Check sheet for the modelled part. Datum: model origin and axes. Units: mm. Face numbers are marked on the shaded views. A direction names the side the tool comes from. Coordinates: 2 decimals unless noted, no trailing zeros. Loops run counter-clockwise (first coordinate to the right, second up) from the corner with the lowest first, then second, coordinate; pieces in that order, holes last. Notation, with made-up numbers: M 2,-8.5 L 27,-8.5 A31 ccw 27,18.5 Z; hole C 82,44 d1. An arc over 180 degrees is marked long. Write each question's results on one line, items separated by ' | '. Start each with the question number.
from build123d import *

# Parameters (mm, degrees)
SKETCH1_W           = 32
SKETCH1_H           = 46
BOSS_EXTRUDE1_DEPTH = 25.2
BOSS_EXTRUDE2_START = 25.2
BOSS_EXTRUDE2_DEPTH = 16.5
SKETCH2_R           = 12.2
BOSS_EXTRUDE3_DEPTH = 30.8


with BuildPart() as part:
    # Sketch1 → Boss-Extrude1 (new body)
    # profile 1 of 2: a face of its own
    with BuildSketch(Plane(origin=(0, 0, 0), x_dir=(1, 0, 0), z_dir=(0, 1, 0))):
        with Locations((0, -8)):
            Rectangle(SKETCH1_W, SKETCH1_H)
        with BuildLine():
            ThreePointArc((-1.8, 2.4), (0, -3), (1.8, 2.4))
            Line((1.8, 2.4), (-1.8, 2.4))
        make_face(mode=Mode.SUBTRACT)
    # profile 2 of 2: a face of its own
    with BuildSketch(Plane(origin=(0, 0, 0), x_dir=(1, 0, 0), z_dir=(0, 1, 0))):
        with BuildLine():
            Line((-1.8, 2.4), (1.8, 2.4))
            ThreePointArc((1.8, 2.4), (0, -3), (-1.8, 2.4))
        make_face()
    extrude(amount=BOSS_EXTRUDE1_DEPTH)

    # Sketch1<3> → Boss-Extrude2 (add)
    with BuildSketch(Plane(origin=(0, 0, 0), x_dir=(1, 0, 0), z_dir=(0, 1, 0)).offset(BOSS_EXTRUDE2_START)):
        with BuildLine():
            Line((-1.8, 2.4), (1.8, 2.4))
            ThreePointArc((1.8, 2.4), (0, -3), (-1.8, 2.4))
        make_face()
    extrude(amount=BOSS_EXTRUDE2_DEPTH)

    # Sketch2 → Boss-Extrude3 (add)
    with BuildSketch(Plane.XY.offset(31)):
        with Locations((3.8, 13)):
            Circle(SKETCH2_R)
    extrude(amount=BOSS_EXTRUDE3_DEPTH)


solid = part.part
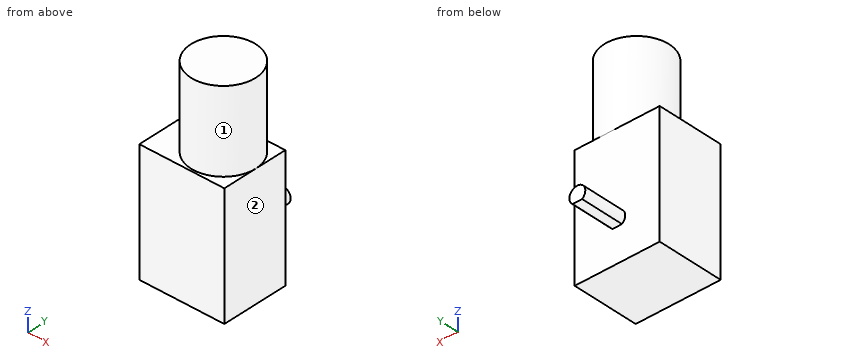
Item 1: Thickness scan on line 1 (Z direction, x = -4, y = 3.5); line 2 (Y direction, x = -2, z = 4); line 3 (Z direction, x = 0.5, y = 40). Record the ranges inside material, lowest first.
Item 2: Section check B-B (y = 4). Record the cut outline in (x, z), plus the area to 3 significant figures.
Item 3: Section check D-D (x = 0). Record the cut outline in (y, z), plus the area to 3 significant figures.
Item 4: Section check A-A (x = 8.5). Record the cut outline in (y, z), plus the area to 3 significant figures.
Item 5: Section check C-C (z = -8). Record the cut outline in (x, y), plus the area to 3 significant figures.
Item 6: Depth check by flat-ended pin: P1, Ø8, axis at x = 3.5, y = 29.5, coming from the -Z side; P2, Ø12, axis at y = 29, z = 47.5, coming from the -X side; P3, Ø1, axis at y = 20, z = 52.5, coming from the +X side; P4, Ø3, axis at y = 28, z = 7, coming from the +X side. Enter the tip coordinate at first touch or a pass-through.
Item 7: Tool access check on the marked faces 1 and 2. Record the directions out of +Z, -Z, +X, -X, +Y, -Y that give a thin tool (end or side, any length) a straight path to the whole face; none if there is none.
Computed values:
1) line 1: z = -15 to 31 | line 2: y = 0 to 25.2 | line 3: z = -2.4 to 2.96
2) outline: M -16,-15 L 16,-15 L 16,31 L 12.04,31 L 12.04,61.8 L -4.44,61.8 L -4.44,31 L -16,31 Z | area: 1,980 mm²
3) outline: M 0,-15 L 25.2,-15 L 25.2,-2.4 L 41.7,-2.4 L 41.7,3 L 25.2,3 L 25.2,31 L 24.59,31 L 24.59,61.8 L 1.41,61.8 L 1.41,31 L 0,31 Z | area: 1,960 mm²
4) outline: M 0,-15 L 25.2,-15 L 25.2,31 L 24.26,31 L 24.26,61.8 L 1.74,61.8 L 1.74,31 L 0,31 Z | area: 1,850 mm²
5) outline: M -16,0 L 16,0 L 16,25.2 L -16,25.2 Z | area: 806 mm²
6) P1: stops at z = -2.4 | P2: stops at x = -3.19 | P3: stops at x = 14.12 | P4: passes through
7) face 1: +Z | face 2: +Z, -Z, +X, +Y, -Y
